```python
from build123d import *

# Parameters (mm, degrees)
SKETCH1_W            = 79.1
SKETCH1_H            = 60
BOSS_EXTRUDE1_DEPTH  = 5
BOSS_EXTRUDE2_DEPTH  = 24
MIRROR2_COPY_1_DEPTH = 24
SKETCH10_R           = 1.55
CUT_EXTRUDE7_DEPTH   = 8
SKETCH11_R           = 3
CUT_EXTRUDE8_DEPTH   = 1
SKETCH12_W           = 27.78460969
SKETCH12_H           = 17.653
SKETCH12_R           = 1.5
SKETCH12_R_2         = 8.15
BOSS_EXTRUDE5_DEPTH  = 10
SKETCH13_W           = 34
SKETCH13_H           = 28
CUT_EXTRUDE9_DEPTH   = 10
FILLET2_R            = 3
SKETCH15_W           = 6
SKETCH15_H           = 2.8
CUT_EXTRUDE12_DEPTH  = 8.2


with BuildPart() as part:
    # Sketch1 → Boss-Extrude1 (new body)
    with BuildSketch(Plane(origin=(0, 0, 0), x_dir=(1, 0, 0), z_dir=(0, 1, 0))):
        Rectangle(SKETCH1_W, SKETCH1_H)
    extrude(amount=BOSS_EXTRUDE1_DEPTH)

    # Sketch2 → Boss-Extrude2 (add)
    with BuildSketch(Plane.XY.offset(30)):
        with BuildLine():
            Line((-39.55, 13.55), (-39.55, 5))
            Line((-39.55, 5), (-20.45, 5))
            Line((-20.45, 5), (-20.45, 13.55))
            Line((-20.45, 13.55), (-22.45, 13.55))
            ThreePointArc((-22.45, 13.55), (-30, 6), (-37.55, 13.55))
            Line((-37.55, 13.55), (-39.55, 13.55))
        make_face()
    boss_extrude2 = extrude(amount=-BOSS_EXTRUDE2_DEPTH)

    # Mirror1: Boss-Extrude2 across plane
    add(boss_extrude2.mirror(Plane.XY))

    # Mirror2: Boss-Extrude2 across plane
    add(boss_extrude2.mirror(Plane(origin=(0, 0, 0), x_dir=(0, 0, 1), z_dir=(1, 0, 0))))

    # Mirror2 copy 1 sketch → Mirror2 copy 1 (add)
    with BuildSketch(Plane(origin=(0, 0, -30), x_dir=(-1, 0, 0), z_dir=(0, 0, -1))):
        with BuildLine():
            Line((-39.55, 13.55), (-39.55, 5))
            Line((-39.55, 5), (-20.45, 5))
            Line((-20.45, 5), (-20.45, 13.55))
            Line((-20.45, 13.55), (-22.45, 13.55))
            ThreePointArc((-22.45, 13.55), (-30, 6), (-37.55, 13.55))
            Line((-37.55, 13.55), (-39.55, 13.55))
        make_face()
    extrude(amount=-MIRROR2_COPY_1_DEPTH)

    # Sketch10 → Cut-Extrude7 (cut)
    with BuildSketch(Plane(origin=(0, 5, 0), x_dir=(1, 0, 0), z_dir=(0, 1, 0))):
        with Locations(Location((-15.45, -26, 0), (0, 0, 270))):
            Circle(SKETCH10_R)
        with Locations(Location((-15.45, 26, 0), (0, 0, 270))):
            Circle(SKETCH10_R)
        with Locations(Location((15.45, 26, 0), (0, 0, 270))):
            Circle(SKETCH10_R)
        with Locations(Location((15.45, -26, 0), (0, 0, 270))):
            Circle(SKETCH10_R)
    extrude(amount=-CUT_EXTRUDE7_DEPTH, mode=Mode.SUBTRACT)

    # Sketch11 → Cut-Extrude8 (cut)
    with BuildSketch(Plane.XZ):
        with Locations(Location((-15.45, 26, 0), (0, 0, 270))):
            Circle(SKETCH11_R)
        with Locations(Location((15.45, 26, 0), (0, 0, 270))):
            Circle(SKETCH11_R)
        with Locations(Location((15.45, -26, 0), (0, 0, 270))):
            Circle(SKETCH11_R)
        with Locations(Location((-15.45, -26, 0), (0, 0, 270))):
            Circle(SKETCH11_R)
    extrude(amount=-CUT_EXTRUDE8_DEPTH, mode=Mode.SUBTRACT)

    # Sketch12 → Boss-Extrude5 (add)
    with BuildSketch(Plane.XY.offset(-10)):
        with Locations((0, -8.8265)):
            Rectangle(SKETCH12_W, SKETCH12_H)
        with Locations(Location((-10.392304845, -14.153, 0), (0, 0, 180))):
            Circle(SKETCH12_R, mode=Mode.SUBTRACT)
        with Locations(Location((10.392304845, -14.153, 0), (0, 0, 180))):
            Circle(SKETCH12_R, mode=Mode.SUBTRACT)
        with Locations(Location((0, -8.153, 0), (0, 0, 180))):
            Circle(SKETCH12_R_2, mode=Mode.SUBTRACT)
    extrude(amount=-BOSS_EXTRUDE5_DEPTH)

    # Sketch13 → Cut-Extrude9 (cut)
    with BuildSketch(Plane.XZ):
        with Locations((0, 4)):
            Rectangle(SKETCH13_W, SKETCH13_H)
    extrude(amount=-CUT_EXTRUDE9_DEPTH, mode=Mode.SUBTRACT)

    # Fillet2
    fillet2_edges = [part.edges().sort_by_distance(p)[0] for p in [
        (-13.892304845, 0, -15),
        (13.892304845, 0, -15),
    ]]
    fillet(fillet2_edges, radius=FILLET2_R)

    # Sketch15 → Cut-Extrude12 (cut)
    with BuildSketch(Plane(origin=(-15.772652423, -15.772652423, 0), x_dir=(-0.7071067811865477, 0.7071067811865475, 0), z_dir=(-0.7071067811865475, -0.7071067811865477, 0))):
        with Locations((-2.659213046, 13.9)):
            Rectangle(SKETCH15_W, SKETCH15_H)
    cut_extrude12 = extrude(amount=-CUT_EXTRUDE12_DEPTH, mode=Mode.SUBTRACT)

    # Mirror3: Cut-Extrude12 across plane
    add(cut_extrude12.mirror(Plane(origin=(0, 0, 0), x_dir=(0, 0, 1), z_dir=(1, 0, 0))), mode=Mode.SUBTRACT)


solid = part.part
```
Work out the finished part from the listing and answer in its coordinate system (mm). A direction names the side the tool comes from. Give positions to 0.01 mm unless a question says otherwise; leave off trailing zeros. Loops run counter-clockwise (first coordinate to the right, second up) from the corner with the lowest first, then second, coordinate; pieces in that order, holes last. Notation, with made-up numbers: (77, 22) - (121, 22) arc R31 cw to (121, 60) - close; hole circle Ø8 at (53.5, 43.25). An arc over 180 degrees is marked (long way). Use CSV: the item, a comma, the result in double quotes. Start each with the question number.
(1) Find the intervals of material crossed by L1, parallel to X at y = 3, z = 26; L2, parallel to Y at x = 0, z = -15.25; L3, parallel to Z at x = 34, y = 6, in increasing order.
(2) Find section D-D, the plane z = 22. Determine the outline of the cut face in (x, y), plus the area to 3 significant figures.
(3) Find section A-A, the plane x = 0. Count the separate pieces of the cut face and the enclosed holes in it, plus the area to 3 significant figures.
(4) Each of these flat-tipped pins is pushed along its axis until it touches: pin 1 (11 mm diameter, centred on y = -11, z = -14, fed in from +X); pin 2 (5 mm diameter, centred on x = -30, z = 22, fed in from -Y); pin 3 (3.5 mm diameter, centred on x = -15.45, z = 26, fed in from -Y); pin 4 (12 mm diameter, centred on y = -9.5, z = 2.5, fed in from -X). Where does it stop, or does it pass through?
(5) Find section B-B, the plane z = 4.5. Determine the outline of the cut face in (x, y).
(6) Determine the mould class of faces 1 (the face through (14.79, -0.86, -15.07)), 2 (the face through (1, 4, 30)), 3 (the face through (-39, 13.55, -18)), 4 (the face through (-10, -16, -12.5)) for opening direction Y: released by +Y, released by -Y, zero draft, split by the parting line, or undercut.
(7) Find section C-C, the plane y = -4. Determine the outline of the cut face in (x, z).
(8) A tool of negligible diameter and unlimited length cuts with its end or side. For faces 5 (the face through (-10, -16, -15.3)), 6 (the face through (-7.837, -15.84, -13.88)), 7 (the face through (13.892, -10, -15)), 8 (the face through (0, -17, -20)), 9 (the face through (30.1, 5.5, -6)), from which of +Z, -Z, +X, -X, +Y, -Y can it reach the whole face along a straight path? Write none if from no direction.
Results found:
1,L1,"-39.55 to -17, -13.9 to 13.9, 17 to 39.55"
1,L2,"-17.65 to -16.3, 0 to 5"
1,L3,"-30 to -6, 6 to 30"
2,outline,"(-39.55, 0) - (39.55, 0) - (39.55, 13.55) - (37.55, 13.55) arc R7.55 cw to (22.45, 13.55) - (20.45, 13.55) - (20.45, 5) - (-20.45, 5) - (-20.45, 13.55) - (-22.45, 13.55) arc R7.55 cw to (-37.55, 13.55) - (-39.55, 13.55) - close"
2,area,"543 mm^2"
3,separate pieces,"3"
3,enclosed holes,"0"
3,area,"174 mm^2"
4,pin 1,"x = 13.89"
4,pin 2,"y = 0"
4,pin 3,"y = 1"
4,pin 4,"through"
5,outline,"(-39.55, 0) - (-17, 0) - (-17, 5) - (-39.55, 5) - close; (17, 0) - (39.55, 0) - (39.55, 5) - (17, 5) - close"
6,face 1,"released by -Y"
6,face 2,"zero draft"
6,face 3,"released by +Y"
6,face 4,"undercut"
7,outline,"(-13.89, -20) - (-7.01, -20) - (-7.01, -10) - (-13.89, -10) - close; (7.01, -20) - (13.89, -20) - (13.89, -10) - (7.01, -10) - close"
8,face 5,"none"
8,face 6,"-X"
8,face 7,"+Z, -Z, +X, -Y"
8,face 8,"-Z, +X, -X, -Y"
8,face 9,"+X, -X, +Y"
